Could you check a few things on this model? Use its own coordinates, in mm. Coordinates: 2 decimals unless noted, no trailing zeros. Loops run counter-clockwise (first coordinate to the right, second up) from the corner with the lowest first, then second, coordinate; pieces in that order, holes last. Notation, with made-up numbers: (10, 58.5) - (22, 58.5) arc R32 cw to (22, 97.5) - close; hole circle Ø8 at (-31, 15.5). An arc over 180 degrees is marked (long way). One line per question, with ' | ' between items. Start each with the question number.
1. I'm going to push a flat-ended pin straight in: P1, Ø2, axis at y = 2, z = -14, coming from the -X side. Where does the tip first touch, or does it pass through?
2. I want a section at A-A, the plane z = -9. Write out the boundary of the cut face in (x, y).
3. We'd pull the mould along X, two halves only. Please class faces 1 (the flat face through (46, 3, -18)), 2 (the cylindrical face through (42.6, 3, -5.8)), 3 (the cylindrical face through (-9, 3, -9)): pulls with the +X half, pulls with the -X half, needs draft (parallel to the pull), parting line crosses it, or undercut.
4. I want a section at B-B, the plane x = 45. Write out the boundary of the cut face in (y, z).
5. I want a section at C-C, the plane y = 1.8. Write out the boundary of the cut face in (x, z).
6. Please list where these lines run through material, in increasing order: L1, parallel to X at y = 3.45, z = -9; L2, parallel to X at y = 3, z = -7.25; L3, parallel to Z at x = 90, y = 3.3. Write a range as [from, to].
7. I want a section at D-D, the plane z = -3.25. Write out the boundary of the cut face in (x, y), then the cut area to 3 significant figures.
from build123d import *

# Parameters (mm, degrees)
BOSS_EXTRUDE1_DEPTH = 6
SKETCH3_R           = 4
CUT_EXTRUDE1_DEPTH  = 6


with BuildPart() as part:
    # Sketch2 → Boss-Extrude1 (new body)
    with BuildSketch(Plane(origin=(0, 0, 0), x_dir=(1, 0, 0), z_dir=(0, 1, 0))):
        with BuildLine():
            Line((0, 0), (90, 0))
            ThreePointArc((90, 0), (99, 9), (90, 18))
            Line((90, 18), (0, 18))
            ThreePointArc((0, 18), (-9, 9), (0, 0))
        make_face()
    extrude(amount=BOSS_EXTRUDE1_DEPTH)

    # Sketch3 → Cut-Extrude1 (cut)
    with BuildSketch(Plane.XZ):
        with Locations(Location((0, -9, 0), (0, 0, 270))):
            Circle(SKETCH3_R)
        with Locations(Location((90, -9, 0), (0, 0, 90))):
            Circle(SKETCH3_R)
        with Locations(Location((45, -9, 0), (0, 0, 270))):
            Circle(SKETCH3_R)
    extrude(amount=-CUT_EXTRUDE1_DEPTH, mode=Mode.SUBTRACT)


solid = part.part
Results are:
1) P1: stops at x = -8.06
2) outline: (-9, 0) - (-4, 0) - (-4, 6) - (-9, 6) - close; (4, 0) - (41, 0) - (41, 6) - (4, 6) - close; (49, 0) - (86, 0) - (86, 6) - (49, 6) - close; (94, 0) - (99, 0) - (99, 6) - (94, 6) - close
3) face 1: needs draft | face 2: undercut | face 3: pulls with the -X half
4) outline: (0, -18) - (6, -18) - (6, -13) - (0, -13) - close; (0, -5) - (6, -5) - (6, 0) - (0, 0) - close
5) outline: (0, -18) - (90, -18) arc R9 ccw to (90, 0) - (0, 0) arc R9 ccw to start; hole circle Ø8 at (0, -9); hole circle Ø8 at (45, -9); hole circle Ø8 at (90, -9)
6) L1: x = [-9, -4], [4, 41], [49, 86], [94, 99] | L2: x = [-8.83, -3.6], [3.6, 41.4], [48.6, 86.4], [93.6, 98.83] | L3: z = [-18, -13], [-5, 0]
7) outline: (-6.92, 0) - (96.92, 0) - (96.92, 6) - (-6.92, 6) - close | area: 623 mm2
